The listing builds one solid part. Answer for the finished solid, in the listing's coordinates (mm). Face numbers are marked on the shaded views. A direction names the side the tool comes from. Give positions to 0.01 mm unless a question says otherwise; leave off trailing zeros. Loops run counter-clockwise (first coordinate to the right, second up) from the corner with the lowest first, then second, coordinate; pieces in that order, holes last.
Item 1: A tool of negligible diameter and unlimited length cuts with its end or side. For the marked faces 1, 2 and 3, from which of +Z, -Z, +X, -X, +Y, -Y can it reach the whole face along a straight path? Write none if from no direction.
Item 2: Section A-A, the plane y = 0 is taken. Give the vertices of the cut face in (x, z), and give its area (3 significant figures).
Item 3: Section C-C, the plane z = 0.3 is taken. Give the vertices of the cut face in (x, y).
Item 4: Consider line 1 along Y through (x, z) = (0, 0.55); line 2 along Z through (x, y) = (3.75, 0.5); line 3 along Y through (x, z) = (8.5, 0.9). Determine where each line is inside the solid, lowest interval first.
Item 5: Section B-B, the plane x = 0 is taken. Give the vertices of the cut face in (y, z), and give its area (3 significant figures).
Item 6: Section D-D, the plane y = -4.5 is taken. Give the vertices of the cut face in (x, z), and give its area (3 significant figures).
Item 7: Each of these flat-tipped pins is pushed along its axis until it touches: pin 1 Ø0.6 at (y, z) = (2.5, 1) entering from -X; pin 2 Ø1 at (y, z) = (1, 1.5) entering from -X; pin 3 Ø1.4 at (x, y) = (-0.5, 6.5) entering from -Z. Where does it stop, or does it pass through?
Solid Edge part; units mm, degrees
sketch "Sketch1" plane through (0, 0, 0) normal (0, 0, 1) x (1, 0, 0)
  circle A0 centre (0, 0) radius 0.5
  circle A1 centre (0, 0) radius 0.75
extrude "Protrusion1" add sketch "Sketch1" along normal up to vertex (0.75 mm away)
sketch "Sketch2" plane through (0, 0, 0.75) normal (0, 0, 1) x (1, 0, 0)
  arc A0 (8.8206, -1.3061) -> (6.6621, -5.9268) centre (7.7413, -3.6164) ccw
  line L0 (6.6621, -5.9268) -> (11.1921, -8.043)
  arc A1 (11.1921, -8.043) -> (13.3507, -3.4223) centre (12.2714, -5.7327) ccw
  line L1 (13.3507, -3.4223) -> (8.8206, -1.3061)
  circle A2 centre (0, 0) radius 0.5
  line L2 (13.647, -2.7881) -> (9.1169, -0.6719)
  arc A3 (9.1169, -0.6719) -> (8.4847, -0.4526) centre (7.7413, -3.6164) ccw
  line L3 (8.4847, -0.4526) -> (0.9584, 1.3157)
  line L4 (0.9584, 1.3157) -> (0.9584, 6)
  line L5 (0.9584, 6) -> (1.5, 7.5)
  line L6 (-1.5, 7.5) -> (1.5, 7.5)
  line L7 (-1.5, 7.5) -> (-0.9416, 6)
  line L8 (-0.9416, 6) -> (-0.9416, 1.1676)
  line L9 (5.7919, -6.2168) -> (-0.8998, -1.2002)
  line L10 (6.3658, -6.561) -> (10.8958, -8.6772)
  arc A4 (10.8958, -8.6772) -> (13.647, -2.7881) centre (12.2714, -5.7327) ccw
  arc A5 (5.7919, -6.2168) -> (6.3658, -6.561) centre (7.7413, -3.6164) ccw
  arc A6 (-0.9416, 1.1676) -> (-0.8998, -1.2002) centre (0, 0) ccw
  dimension "D1" = 6.3658
  dimension "D2" = 1.5
extrude "Protrusion2" add sketch "Sketch2" along normal blind 0.5
sketch "Sketch3" plane through (0, 0, 1.25) normal (0, 0, 1) x (1, 0, 0)
  line L0 (1.5, 7.5) -> (-1.5, 7.5)
  line L1 (-1.5, 7.5) -> (-0.9416, 6)
  line L2 (-0.9416, 6) -> (-0.9416, 3)
  line L3 (-0.9416, 3) -> (0.9584, 3)
  line L4 (0.9584, 3) -> (0.9584, 6)
  line L5 (0.9584, 6) -> (1.5, 7.5)
extrude "ExtrudedProtrusion_3" add sketch "Sketch3" along normal blind 1.5
sketch "Sketch4" plane through (0.9584, 5.4372, 2.375) normal (1, 0, 0) x (0, 1, 0)
  line L0 (-2.4372, -1.125) -> (-1.3869, 0.375)
  line L1 (-2.4372, 1.625) -> (-2.4372, -1.125)
extrude "Cutout1" cut sketch "Sketch4" against normal through all material side at (0.9584, 3.4842, 2.0287)
sketch "Sketch5" plane through (0.9584, 5.4372, 2.375) normal (1, 0, 0) x (0, 1, 0)
  line L0 (-2.0276, -1.4118) -> (-1.1266, -0.125)
  line L1 (-1.1266, -0.125) -> (-0.4372, -0.125)
extrude "Cutout2" cut sketch "Sketch5" along normal through all and the other way through all material side at (0.9584, 3.9011, 1.5779)
fillet "Round_1" radius 0.25 2 edges at (1.5, 7.5, 2.5) (-1.5, 7.5, 2.5)
properties material "Polypropylene, high impact"
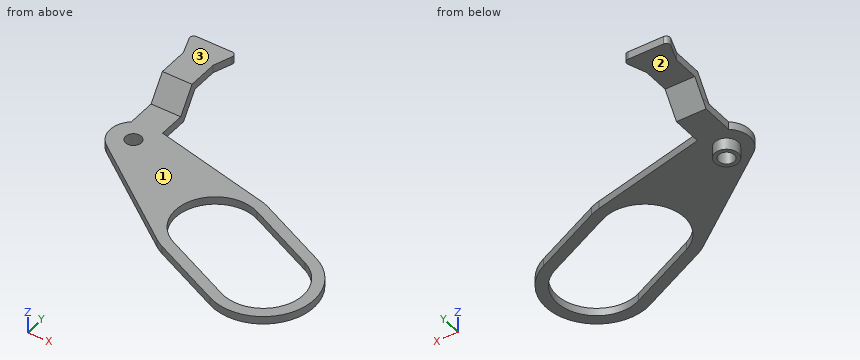
Worked answers:
1. face 1: +Z, +X, -X, -Y
1. face 2: -Z, +X, -X, +Y
1. face 3: +Z, +X, -X, +Y, -Y
2. outline: (-1.5, 0.75) - (-0.75, 0.75) - (-0.75, 0) - (-0.5, 0) - (-0.5, 1.25) - (-1.5, 1.25) - close; (0.5, 0) - (0.75, 0) - (0.75, 0.75) - (6.56, 0.75) - (6.56, 1.25) - (0.5, 1.25) - close
2. area: 3.90 mm2
3. outline: circle Ø1.5 at (0, 0); hole circle Ø1 at (0, 0)
4. line 1: y = -0.75 to -0.5, 0.5 to 0.75
4. line 2: z = 0.75 to 1.25
4. line 3: y = -7.56 to -6.79, -1.18 to -0.46
5. outline: (-1.87, 0.75) - (-0.75, 0.75) - (-0.75, 0) - (-0.5, 0) - (-0.5, 1.25) - (-1.87, 1.25) - close; (0.5, 0) - (0.75, 0) - (0.75, 0.75) - (3.26, 0.75) - (4.31, 2.25) - (7.5, 2.25) - (7.5, 2.75) - (4.05, 2.75) - (3, 1.25) - (0.5, 1.25) - close
5. area: 4.95 mm2
6. outline: (3.5, 0.75) - (5.35, 0.75) - (5.35, 1.25) - (3.5, 1.25) - close; (14.5, 0.75) - (15.28, 0.75) - (15.28, 1.25) - (14.5, 1.25) - close
6. area: 1.31 mm2
7. pin 1: stops at x = -0.94
7. pin 2: stops at x = -1.39
7. pin 3: stops at z = 2.25
